from build123d import *

# Parameters (mm, degrees)
F0_W      = 92
F0_H      = 56
F1_DEPTH  = 1.5
F2_W      = 2
F2_H      = 56
F3_DEPTH  = 4
F5_W      = 92
F5_H      = 2
F6_DEPTH  = 4
F8_W      = 2
F8_H      = 56
F9_DEPTH  = 4
F11_W     = 2
F11_H     = 56
F12_DEPTH = 4
F14_W     = 92
F14_H     = 2
F15_DEPTH = 4


# Not quite as in the source:
# - a feature names something its author has since deleted; it is built from what else it names


with BuildPart() as f1:
    # F0 (on Top) → F1 (new body)
    with BuildSketch(Plane.XY):
        Rectangle(F0_W, F0_H)
    extrude(amount=F1_DEPTH)

    # F4: F3 across plane


with BuildPart() as f3:
    # F2 (on Top) → F3 (new body)
    with BuildSketch(Plane.XY):
        with Locations((45, 0)):
            Rectangle(F2_W, F2_H)
    extrude(amount=F3_DEPTH)


with BuildPart() as f1_1:
    add(f1.part)
    add(f3.part.mirror(Plane.YZ))


    add(f3.part)  # F6 merges F3
    # F5 (on Top) → F6 (join)
    with BuildSketch(Plane.XY):
        with Locations((0, -27)):
            Rectangle(F5_W, F5_H)
    extrude(amount=F6_DEPTH)

    # F7: F1 across plane


with BuildPart() as f1_2:
    add(f1_1.part)
    add(f1_1.part.mirror(Plane.XZ))

    # F8 (on Top) → F9 (join)
    with BuildSketch(Plane.XY):
        with Locations((27, 0)):
            Rectangle(F8_W, F8_H)
    extrude(amount=F9_DEPTH)

    # F10: F1 across plane


with BuildPart() as f1_3:
    add(f1_2.part)
    add(f1_2.part.mirror(Plane.YZ))

    # F11 (on Top) → F12 (join)
    with BuildSketch(Plane.XY):
        with Locations((9, 0)):
            Rectangle(F11_W, F11_H)
    extrude(amount=F12_DEPTH)

    # F13: F1 across plane


with BuildPart() as f1_4:
    add(f1_3.part)
    add(f1_3.part.mirror(Plane.YZ))

    # F14 (on Top) → F15 (join)
    with BuildSketch(Plane.XY):
        Rectangle(F14_W, F14_H)
    extrude(amount=F15_DEPTH)


solid = f1_4.part
The listing builds one solid part. Answer for the finished solid, in the listing's coordinates (mm). Give positions to 0.01 mm unless a question says otherwise; leave off trailing zeros. Loops run counter-clockwise (first coordinate to the right, second up) from the corner with the lowest first, then second, coordinate; pieces in that order, holes last.
Item 1: A cutting plane is placed at C-C (z = 2.7). Give the number of separate pieces and of enclosed holes in the cut face, then the cut area to 3 significant figures.
Derived:
separate pieces: 1
enclosed holes: 10
area: 1,150 mm2
Item 2: Find the intervals of material crossed by line 1 along Y through (x, z) = (20.5, 1.75); line 2 along X through (y, z) = (9, 3.2); line 3 along Z through (x, y) = (35.5, 17), in increasing order.
Derived:
line 1: y = -28 to -26, -1 to 1, 26 to 28
line 2: x = -46 to -44, -28 to -26, -10 to -8, 8 to 10, 26 to 28, 44 to 46
line 3: z = 0 to 1.5
Item 3: A cutting plane is placed at A-A (y = 5.5). Give the vertices of the cut face in (x, z).
Derived:
outline: (-46, 0) - (46, 0) - (46, 4) - (44, 4) - (44, 1.5) - (28, 1.5) - (28, 4) - (26, 4) - (26, 1.5) - (10, 1.5) - (10, 4) - (8, 4) - (8, 1.5) - (-8, 1.5) - (-8, 4) - (-10, 4) - (-10, 1.5) - (-26, 1.5) - (-26, 4) - (-28, 4) - (-28, 1.5) - (-44, 1.5) - (-44, 4) - (-46, 4) - close
Item 4: This flat-tipped pin is pushed along its axis until it touches: pin 1 Ø3 at (x, y) = (-33, -15.5) entering from +Z. Where does it stop, or does it pass through?
Derived:
pin 1: stops at z = 1.5
Item 5: A cutting plane is placed at B-B (x = -12.5). Give the vertices of the cut face in (y, z).
Derived:
outline: (-28, 0) - (28, 0) - (28, 4) - (26, 4) - (26, 1.5) - (1, 1.5) - (1, 4) - (-1, 4) - (-1, 1.5) - (-26, 1.5) - (-26, 4) - (-28, 4) - close
Item 6: Determine the mould class of faces 1 (the flat face through (0, -1, 3)), 2 (the flat face through (-1, -28, 2)), 3 (the flat face through (46, 0, 2)) for opening direction X: +X half, -X half, draft (parallel to the pull), parting line (faces both ways), or undercut.
Derived:
face 1: undercut
face 2: draft
face 3: +X half
